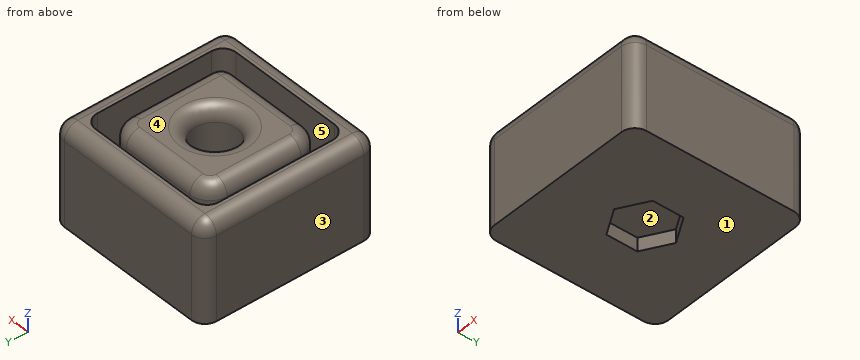
Autodesk Inventor part; units mm, degrees
ref_plane "YZ Plane" through (0, 0, 0) normal (1, 0, 0) x (0, 1, 0)
ref_plane "XZ Plane" through (0, 0, 0) normal (0, 1, 0) x (-1, 0, 0)
ref_plane "XY Plane" through (0, 0, 0) normal (0, 0, 1) x (1, 0, 0)
sketch "Schizzo1" plane through (0, 0, 0) normal (0, 0, 1) x (1, 0, 0)
  line L0 (6.5, -8.5) -> (-5.5, -8.5)
  line L1 (-8.5, -5.5) -> (-8.5, 5.5)
  line L2 (-5.5, 8.5) -> (5.5, 8.5)
  line L3 (8.5, 5.5) -> (8.5, -6.5)
  arc A0 (6.5, -8.5) -> (8.5, -6.5) centre (6.5, -6.5) ccw
  arc A1 (-8.5, -5.5) -> (-5.5, -8.5) centre (-5.5, -5.5) ccw
  arc A2 (-5.5, 8.5) -> (-8.5, 5.5) centre (-5.5, 5.5) ccw
  arc A3 (8.5, 5.5) -> (5.5, 8.5) centre (5.5, 5.5) ccw
  point P0 (0, 0)
  point P1 (0, 0)
  point P2 (8.5, -8.5)
  point P3 (-8.5, -8.5)
  point P4 (-8.5, 8.5)
  point P5 (8.5, 8.5)
  dimension "d0" = 17
  dimension "d44" = 2
  dimension "d45" = 3
extrude "Estrusione1" add sketch "Schizzo1" along normal blind 10
sketch "Schizzo2" plane through (0, 0, 0) normal (0, 0, -1) x (-1, 0, 0)
  line L0 (11, -13) -> (-11, -13)
  line L1 (-13, -11) -> (-13, 11)
  line L2 (-11, 13) -> (11, 13)
  line L3 (13, 11) -> (13, -11)
  line L4 (13, -13) -> (-13, 13) construction
  line L5 (-13, -13) -> (13, 13) construction
  arc A0 (13, 11) -> (11, 13) centre (11, 11) ccw
  arc A1 (11, -13) -> (13, -11) centre (11, -11) ccw
  arc A2 (-13, -11) -> (-11, -13) centre (-11, -11) ccw
  arc A3 (-11, 13) -> (-13, 11) centre (-11, 11) ccw
  point P0 (0, 0)
  dimension "d3" = 26
  dimension "d4" = 26
  dimension "d145" = 2
extrude "Estrusione2" add sketch "Schizzo2" along normal blind 4.5
sketch "Schizzo12" plane through (0, 0, 0) normal (0, 0, 1) x (1, 0, 0)
  line L0 (-10.5, -8.5) -> (-10.5, 8.5)
  line L1 (-8.5, 10.5) -> (8.5, 10.5)
  line L2 (10.5, 8.5) -> (10.5, -8.5)
  line L3 (8.5, -10.5) -> (-8.5, -10.5)
  line L4 (-13, -11) -> (-13, 11)
  line L5 (-11, 13) -> (11, 13)
  line L6 (13, 11) -> (13, -11)
  line L7 (11, -13) -> (-11, -13)
  arc A0 (10.5, 8.5) -> (8.5, 10.5) centre (8.5, 8.5) ccw
  arc A1 (13, 11) -> (11, 13) centre (11, 11) ccw
  arc A2 (11, -13) -> (13, -11) centre (11, -11) ccw
  arc A3 (8.5, -10.5) -> (10.5, -8.5) centre (8.5, -8.5) ccw
  arc A4 (-13, -11) -> (-11, -13) centre (-11, -11) ccw
  arc A5 (-10.5, -8.5) -> (-8.5, -10.5) centre (-8.5, -8.5) ccw
  arc A6 (-11, 13) -> (-13, 11) centre (-11, 11) ccw
  arc A7 (-8.5, 10.5) -> (-10.5, 8.5) centre (-8.5, 8.5) ccw
  point P0 (0, 0)
  point P1 (0, 0)
  point P2 (-10.5, -10.5)
  point P3 (-10.5, 10.5)
  point P4 (10.5, 10.5)
  point P5 (10.5, -10.5)
  point P6 (0, 0)
  point P7 (-13, -13)
  point P8 (-13, 13)
  point P9 (13, 13)
  point P10 (13, -13)
  dimension "d110" = 21
  dimension "d111" = 26
  dimension "d112" = 2
extrude "Estrusione6" add sketch "Schizzo12" along normal blind 10
fillet "Raccordo3" radius 2 1 edges at (0, -13, 10)
fillet "Raccordo8" radius 2 1 edges at (0, 8.5, 10)
sketch "Schizzo20" plane through (0, 0, 10) normal (0, 0, 1) x (1, 0, 0)
  circle A0 centre (0, 0) radius 3.25
  dimension "d176" = 6.5
extrude "Estrusione9" cut sketch "Schizzo20" against normal blind 10
fillet "Raccordo9" radius 2 1 edges at (-3.25, 0, 10)
sketch "Schizzo21" plane through (0, 0, -4.5) normal (0, 0, -1) x (-1, 0, 0)
  circle A0 centre (0, 0) radius 4
  line L0 (-4, 2.3094) -> (0, 4.6188)
  line L1 (0, 4.6188) -> (4, 2.3094)
  line L2 (4, 2.3094) -> (4, -2.3094)
  line L3 (4, -2.3094) -> (0, -4.6188)
  line L4 (0, -4.6188) -> (-4, -2.3094)
  line L5 (-4, -2.3094) -> (-4, 2.3094)
  point P0 (-4, 0)
  dimension "d180" = 8
extrude "Estrusione10" cut sketch "Schizzo21" against normal blind 2
properties part number "2_Connettore_inf_sup"
Could you check a few things on this model? Use its own coordinates, in mm. Face numbers are marked on the shaded views. A direction names the side the tool comes from. Coordinates: 2 decimals unless noted, no trailing zeros. Write each loop counter-clockwise with the first axis right and the second up, starting at its lowest first coordinate (ties: lowest second). Pieces come first, ordered by that corner, then holes. Notation, with made-up numbers: (86, -31.5) - (119, -31.5) arc R12 ccw to (119, -20.5) - close; hole circle Ø7 at (76.25, 81.5). An arc over 180 degrees is marked (long way). Use a Markdown table: item, result.
Q1. Please list where these lines run through material, in increasing order: L1, parallel to Y at x = 0, z = 5.25; L2, parallel to Y at x = 4, z = 2.75.
Geometry check:
| item | result |
|---|---|
| L1 | y = -13 to -10.5, -8.5 to -3.25, 3.25 to 8.5, 10.5 to 13 |
| L2 | y = -13 to -10.5, -8.5 to 8.5, 10.5 to 13 |
Q2. Thinking about a two-plate mould opening in X: for the marked faces 1, 2 and 3, which applies, +X half, -X half, draft (parallel to the pull), parting line (faces both ways), or undercut?
Geometry check:
| item | result |
|---|---|
| face 1 | draft |
| face 2 | undercut |
| face 3 | -X half |
Q3. Imagine slicing it at A-A (z = 4.75). List the corners of the cut face in (x, y) for me, and give its area (3 significant figures).
Geometry check:
| item | result |
|---|---|
| outline | (-13, -11) arc R2 ccw to (-11, -13) - (11, -13) arc R2 ccw to (13, -11) - (13, 11) arc R2 ccw to (11, 13) - (-11, 13) arc R2 ccw to (-13, 11) - close; (-8.5, -5.5) arc R3 ccw to (-5.5, -8.5) - (6.5, -8.5) arc R2 ccw to (8.5, -6.5) - (8.5, 5.5) arc R3 ccw to (5.5, 8.5) - (-5.5, 8.5) arc R3 ccw to (-8.5, 5.5) - close; hole (-10.5, -8.5) arc R2 ccw to (-8.5, -10.5) - (8.5, -10.5) arc R2 ccw to (10.5, -8.5) - (10.5, 8.5) arc R2 ccw to (8.5, 10.5) - (-8.5, 10.5) arc R2 ccw to (-10.5, 8.5) - close; hole circle Ø6.5 at (0, 0) |
| area | 484 mm2 |
Q4. Imagine slicing it at B-B (y = 0). List the corners of the cut face in (x, z) for me, and give its area (3 significant figures).
Geometry check:
| item | result |
|---|---|
| outline | (-13, -4.5) - (-4, -4.5) - (-4, -2.5) - (4, -2.5) - (4, -4.5) - (13, -4.5) - (13, 8) arc R2 ccw to (11, 10) - (10.5, 10) - (10.5, 0) - (8.5, 0) - (8.5, 8) arc R2 ccw to (6.5, 10) - (5.25, 10) arc R2 ccw to (3.25, 8) - (3.25, 0) - (-3.25, 0) - (-3.25, 8) arc R2 ccw to (-5.25, 10) - (-6.5, 10) arc R2 ccw to (-8.5, 8) - (-8.5, 0) - (-10.5, 0) - (-10.5, 10) - (-11, 10) arc R2 ccw to (-13, 8) - close |
| area | 251 mm2 |
Q5. Imagine slicing it at D-D (y = -10). List the corners of the cut face in (x, z) for me, and give its area (3 significant figures).
Geometry check:
| item | result |
|---|---|
| outline | (-13, -4.5) - (13, -4.5) - (13, 8) arc R2 ccw to (11, 10) - (9.82, 10) - (9.82, 0) - (-9.82, 0) - (-9.82, 10) - (-11, 10) arc R2 ccw to (-13, 8) - close |
| area | 179 mm2 |
Q6. Imagine slicing it at C-C (z = -3). List the corners of the cut face in (x, y) for me.
Geometry check:
| item | result |
|---|---|
| outline | (-13, -11) arc R2 ccw to (-11, -13) - (11, -13) arc R2 ccw to (13, -11) - (13, 11) arc R2 ccw to (11, 13) - (-11, 13) arc R2 ccw to (-13, 11) - close; hole (-4, -2.31) - (0, -4.62) - (4, -2.31) - (4, 2.31) - (0, 4.62) - (-4, 2.31) - close |
Q7. Which directions (+Z, -Z, +X, -X, +Y, -Y) give clear straight access to the entire face, cutting with the end or side of a thin tool? Please do the marked faces 4 and 5.
Geometry check:
| item | result |
|---|---|
| face 4 | +Z, +X, -X, +Y, -Y |
| face 5 | +Z |
Q8. I'm going to push a flat-ended pin straight in: pin 1 Ø3 at (x, y) = (-0.5, 1.5) entering from +Z. Where does the tip first touch, or does it pass through?
Geometry check:
| item | result |
|---|---|
| pin 1 | stops at z = 0 |
